Design review of the part built by this model. Coordinates are the model's own, in mm. A direction names the side the tool comes from. Coordinates: 2 decimals unless noted, no trailing zeros. Write each loop counter-clockwise with the first axis right and the second up, starting at its lowest first coordinate (ties: lowest second). Pieces come first, ordered by that corner, then holes. Notation, with made-up numbers: (25, -40) -> (71, -40) arc R16 cw to (71, -28) -> close; hole circle Ø10 at (6.25, -0.5). An arc over 180 degrees is marked (long way). Answer in a Markdown table with one row per item. Add a question column.
Item 1: Take a section at D-D, the plane y = 2. Write out the cut boundary in (x, z), and give its area (3 significant figures).
Item 2: Take a section at C-C, the plane z = -10. Write out the cut boundary in (x, y), and give its area (3 significant figures).
Item 3: Take a section at B-B, the plane x = -5. Write out the cut boundary in (y, z).
Item 4: Draft analysis for pull direction Z (two halves, no side actions). For faces 4 (the face through (5.67, 11.617, -1.479)), 5 (the face through (0.14, 5.301, -5.285)), 6 (the face through (0, 7, 0)), 7 (the face through (-3.45, 1.48, -9.19)), state which applies: released by +Z, released by -Z, zero draft, split by the parting line, or undercut.
Item 5: Clearance check with flat-ended pins moving along their axes: P1, Ø5.5, axis at x = -5, z = -10, coming from the +Y side; P2, Ø6.5, axis at x = 5.5, y = 10.5, coming from the -Z side; P3, Ø5, axis at x = -0.5, z = -13, coming from the +Y side; P4, Ø1.8, axis at x = 4.5, z = -9.5, coming from the +Y side. State where each tip first meets the part, or that it passes through.
Item 6: To check wall thickness, follow line 1 (X direction, y = 4.45, z = -10); line 2 (X direction, y = 10, z = -1.5); line 3 (Y direction, x = 5, z = -4.1). State the ranges of each line that lie inside material, in increasing order.
Item 7: For faces 1 (the face through (0, 10, -5)), 2 (the face through (5, 3, -8)), 3 (the face through (-2.338, 11.384, -3.986)), list the 3-axis set-ups (+Z, -Z, +X, -X, +Y, -Y) from which the entire face can be reached by the end or side of a thin tool; tool diameter is ignored.
Item 8: Take a section at A-A, the plane y = 10. Write out the cut boundary in (x, z).
Autodesk Inventor part; units mm, degrees
ref_plane "YZ Plane" through (0, 0, 0) normal (1, 0, 0) x (0, 1, 0)
ref_plane "XZ Plane" through (0, 0, 0) normal (0, 1, 0) x (-1, 0, 0)
ref_plane "XY Plane" through (0, 0, 0) normal (0, 0, 1) x (1, 0, 0)
sketch "Sketch1" plane through (0, 0, 0) normal (0, 1, 0) x (-1, 0, 0)
  line L0 (10, 0) -> (-10, 0)
  line L1 (10, -5) -> (-10, -5)
  line L2 (-10, 0) -> (-10, -15)
  line L3 (-10, -15) -> (10, -15)
  line L4 (10, -15) -> (10, 0)
  point P0 (0, 0)
  dimension "d15" = 15
  dimension "d16" = 20
extrude "Extrusion1" add sketch "Sketch1" along normal blind 15 contours L4 L1 L2 L0
extrude "Extrusion2" add sketch "Sketch1" along normal blind 5 contours L4 L3 L2 L1
sketch "Sketch2" plane through (0, 5, 0) normal (0, 1, 0) x (1, 0, 0)
  line L0 (-10, 15) -> (-10, 0)
  line L1 (-10, 15) -> (-5, 15)
  line L2 (10, 15) -> (-10, 15)
  line L3 (-5, 15) -> (-5, 10)
  line L4 (10, 15) -> (5, 15)
  line L5 (5, 15) -> (5, 10)
  point P0 (0, 0)
  dimension "d21" = 5
  dimension "d22" = 5
  dimension "d23" = 5
  dimension "d24" = 5
  dimension "d60" = 10
hole "Hole1" at (-5, 5, -10) direction (0, -1, 0) diameter 3.5 end through all counterbore diameter 6 counterbore depth 2
hole "Hole2" at (5, 5, -10) direction (0, -1, 0) diameter 3.5 end through all counterbore diameter 6 counterbore depth 2
sketch "Sketch3" plane through (10, 15, -5) normal (0, 0, -1) x (-1, 0, 0)
  line L0 (20, -10) -> (20, 0)
  line L1 (20, 0) -> (15, 0)
  line L2 (0, 0) -> (20, 0)
  line L3 (15, 0) -> (15, -5)
  line L4 (0, -10) -> (0, 0)
  line L5 (0, 0) -> (5, 0)
  line L6 (5, 0) -> (5, -5)
  point P0 (10, -15)
  dimension "d39" = 5
  dimension "d40" = 5
  dimension "d41" = 5
  dimension "d42" = 5
hole "Hole3" at (-5, 10, -5) direction (0, 0, 1) diameter 3.5 end through all counterbore diameter 6 counterbore depth 2
hole "Hole4" at (5, 10, -5) direction (0, 0, 1) diameter 3.5 end through all counterbore diameter 6 counterbore depth 2
fillet "Fillet2" radius 2 4 edges at (-10, 2.5, -15) (10, 2.5, -15) (10, 15, -2.5) (-10, 15, -2.5)
fillet "Fillet2" radius 1 1 edges at (0, 5, -5)
properties part number "Brackets RC mounting board"
Answers:
| question | item | result |
|---|---|---|
| 1 | outline | (-10, -13) arc R2 ccw to (-8, -15) -> (8, -15) arc R2 ccw to (10, -13) -> (10, 0) -> (-10, 0) -> close; hole circle Ø3.5 at (-5, -10); hole circle Ø3.5 at (5, -10) |
| 1 | area | 279 mm^2 |
| 2 | outline | (-10, 0) -> (-6.75, 0) -> (-6.75, 3) -> (-8, 3) -> (-8, 5) -> (-10, 5) -> close; (-3.25, 0) -> (3.25, 0) -> (3.25, 3) -> (2, 3) -> (2, 5) -> (-2, 5) -> (-2, 3) -> (-3.25, 3) -> close; (6.75, 0) -> (10, 0) -> (10, 5) -> (8, 5) -> (8, 3) -> (6.75, 3) -> close |
| 2 | area | 55.0 mm^2 |
| 3 | outline | (0, -15) -> (5, -15) -> (5, -13) -> (3, -13) -> (3, -11.75) -> (0, -11.75) -> close; (0, -8.25) -> (3, -8.25) -> (3, -7) -> (5, -7) -> (5, -6) arc R1 cw to (6, -5) -> (7, -5) -> (7, -3) -> (8.25, -3) -> (8.25, 0) -> (0, 0) -> close; (11.75, -3) -> (13, -3) -> (13, -5) -> (15, -5) -> (15, 0) -> (11.75, 0) -> close |
| 4 | face 4 | zero draft |
| 4 | face 5 | released by -Z |
| 4 | face 6 | released by +Z |
| 4 | face 7 | undercut |
| 5 | P1 | stops at y = 3 |
| 5 | P2 | stops at z = -5 |
| 5 | P3 | stops at y = 5 |
| 5 | P4 | passes through |
| 6 | line 1 | x = -10 to -8, -2 to 2, 8 to 10 |
| 6 | line 2 | x = -10 to -6.75, -3.25 to 3.25, 6.75 to 10 |
| 6 | line 3 | y = 0 to 7, 13 to 15 |
| 7 | face 1 | -Z, +X, -X, +Y |
| 7 | face 2 | +Y |
| 7 | face 3 | -Z |
| 8 | outline | (-10, -5) -> (-8, -5) -> (-8, -3) -> (-6.75, -3) -> (-6.75, 0) -> (-10, 0) -> close; (-3.25, -3) -> (-2, -3) -> (-2, -5) -> (2, -5) -> (2, -3) -> (3.25, -3) -> (3.25, 0) -> (-3.25, 0) -> close; (6.75, -3) -> (8, -3) -> (8, -5) -> (10, -5) -> (10, 0) -> (6.75, 0) -> close |
